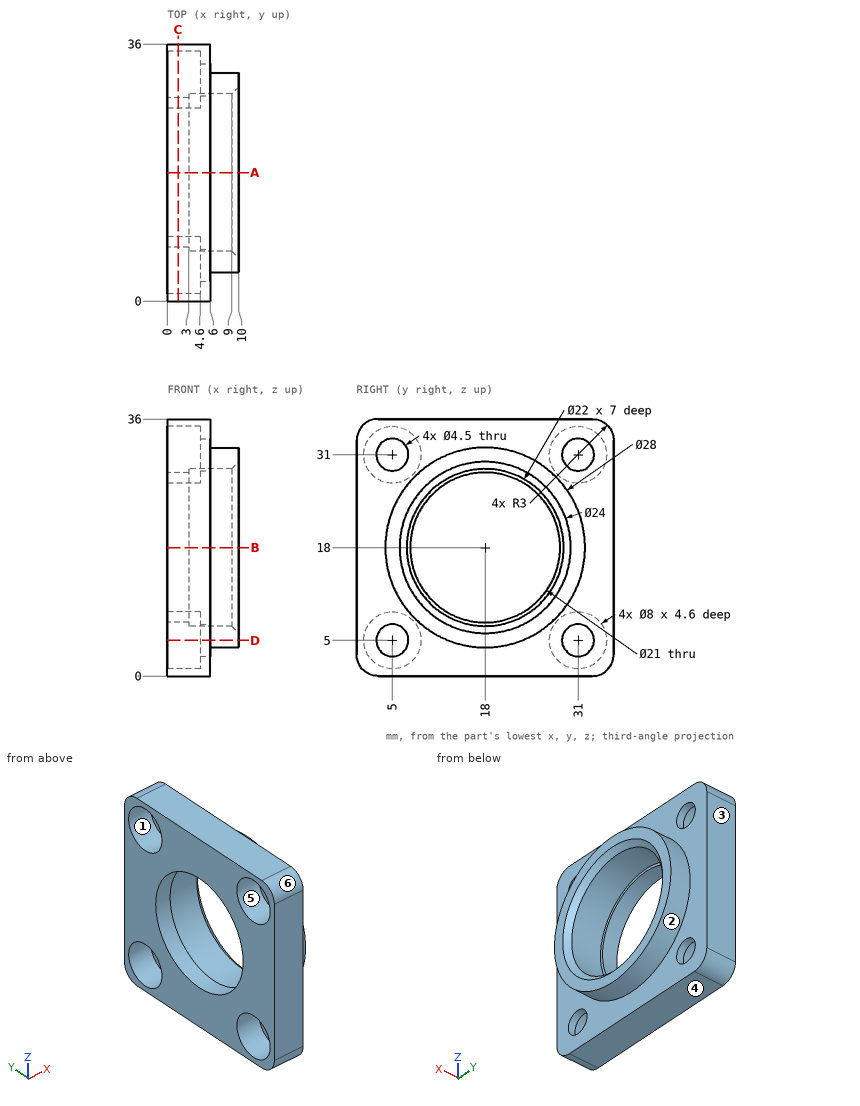
Print and shaded views of the part. All mm, measured from the part's lowest x, y and z. A direction names the side the tool comes from. Give positions to 0.01 mm unless a question says otherwise; leave off trailing zeros. Write each loop counter-clockwise with the first axis right and the second up, starting at its lowest first coordinate (ties: lowest second). Pieces come first, ordered by that corner, then holes. Notation, with made-up numbers: M 13.5,13 L 59.5,13 A9 cw 59.5,27 Z; hole C 42,33.5 d4. An arc over 180 degrees is marked long. Use a Markdown table: item, result.
1) Cut at C-C (x = 1.5). List the corners of the cut face in (y, z).
Responses:
| item | result |
|---|---|
| outline | M 0,3 A3 ccw 3,0 L 33,0 A3 ccw 36,3 L 36,33 A3 ccw 33,36 L 3,36 A3 ccw 0,33 Z; hole C 5,5 d8; hole C 5,31 d8; hole C 18,18 d21; hole C 31,5 d8; hole C 31,31 d8 |
2) Tool access for the marked faces 1, 2 and 3: list every direction of +Z, -Z, +X, -X, +Y, -Y with a clear straight run to the whole face (end or side of a thin tool).
Responses:
| item | result |
|---|---|
| face 1 | -X |
| face 2 | +X |
| face 3 | +Z, -Z, +X, -X, +Y |
3) Drill centre lines: line 1 (Y direction, x = 2.15, z = 31); line 2 (Z direction, x = 0.9, y = 18); line 3 (Y direction, x = 5.4, z = 5). Where is each one in solid material? Low to high. Write a range as from..to.
Responses:
| item | result |
|---|---|
| line 1 | y = 0..1, 9..27, 35..36 |
| line 2 | z = 0..7.5, 28.5..36 |
| line 3 | y = 0..2.75, 7.25..28.75, 33.25..36 |
4) Pin check, flat tips, straight feed: pin 1 (6 mm diameter, centred on y = 5, z = 31, fed in from +X); pin 2 (6 mm diameter, centred on y = 5, z = 5, fed in from -X); pin 3 (17 mm diameter, centred on y = 18, z = 18, fed in from -X); pin 4 (1 mm diameter, centred on x = 7, y = 11.5, fed in from +Z). Stop position of each tip, or through.
Responses:
| item | result |
|---|---|
| pin 1 | stops at x = 6 |
| pin 2 | stops at x = 4.6 |
| pin 3 | passes through |
| pin 4 | stops at z = 30.65 |
5) Cut at A-A (y = 18). List the corners of the cut face in (x, z).
Responses:
| item | result |
|---|---|
| outline | M 0,0 L 6,0 L 6,4 L 10,4 L 10,6 L 9,7 L 3,7 L 3,7.5 L 0,7.5 Z; M 0,28.5 L 3,28.5 L 3,29 L 9,29 L 10,30 L 10,32 L 6,32 L 6,36 L 0,36 Z |
6) Cut at D-D (z = 5). List the corners of the cut face in (x, y).
Responses:
| item | result |
|---|---|
| outline | M 0,0 L 6,0 L 6,2.75 L 4.6,2.75 L 4.6,1 L 0,1 Z; M 0,9 L 4.6,9 L 4.6,7.25 L 6,7.25 L 6,12.8 L 10,12.8 L 10,23.2 L 6,23.2 L 6,28.75 L 4.6,28.75 L 4.6,27 L 0,27 Z; M 0,35 L 4.6,35 L 4.6,33.25 L 6,33.25 L 6,36 L 0,36 Z |
7) Pull direction Y, two halves, no side cores. Call the marked faces 4, 5 and 6: +Y half, -Y half, draft (parallel to the pull), parting line (faces both ways), or undercut.
Responses:
| item | result |
|---|---|
| face 4 | draft |
| face 5 | undercut |
| face 6 | -Y half |
